Part model, mm, in its own coordinate system. Coordinates: 2 decimals unless noted, no trailing zeros. Order: outer loops, then holes, each group sorted by start corner. A loop starts at its lowest first (then second) coordinate and runs counter-clockwise, first axis right, second up.
1) Mould opens along Y. For faces 1 (the flat face through (24, 10, -4)), 2 (the cylindrical face through (64.851, 7.578, -18.437)), 3 (the cylindrical face through (67.67, 5.78, 10.32)), 4 (the flat face through (24, 5, -19.07)) say: +Y half, -Y half, draft (parallel to the pull), parting line (faces both ways), or undercut.
2) Wall check: L1, parallel to X at y = 5, z = -18.7; L2, parallel to X at y = 6.5, z = 3; L3, parallel to Z at x = 62.5, y = 1.5. Give the ranges that are in metal, low to high.
3) Cut at A-A (y = 5). List the corners of the cut face in (x, z), and give its area (3 significant figures).
4) Cut at C-C (z = -15.5). List the corners of the cut face in (x, y).
5) Pin check, flat tip, straight feed: pin 1 Ø7.5 at (x, z) = (65.19, -11.57) entering from -Y. Stop position of the tip, or through.
6) Cut at B-B (z = -9). List the corners of the cut face in (x, y).
```python
from build123d import *

# Parameters (mm, degrees)
SKETCH1_W           = 100
SKETCH1_H           = 30
SKETCH1_R           = 6.45
BOSS_EXTRUDE1_DEPTH = 10
SKETCH2_R           = 2.6
CUT_EXTRUDE1_DEPTH  = 82.56838771


with BuildPart() as part:
    # Sketch1 → Boss-Extrude1 (new body)
    with BuildSketch(Plane(origin=(0, 0, 0), x_dir=(1, 0, 0), z_dir=(0, 1, 0))):
        with Locations((25.189107413, 4.069591528)):
            Rectangle(SKETCH1_W, SKETCH1_H)
        with Locations(Location((65.189107413, 11.569591528, 0), (0, 0, 270))):
            Circle(SKETCH1_R, mode=Mode.SUBTRACT)
        with Locations(Location((65.189107413, -3.430408472, 0), (0, 0, 270))):
            Circle(SKETCH1_R, mode=Mode.SUBTRACT)
    extrude(amount=BOSS_EXTRUDE1_DEPTH)

    # Sketch2 → Cut-Extrude1 (cut, through all)
    with BuildSketch(Plane.XY.offset(10.930408472)):
        with Locations((65.189107413, 5)):
            Circle(SKETCH2_R)
    extrude(amount=-CUT_EXTRUDE1_DEPTH, mode=Mode.SUBTRACT)


solid = part.part
```
Geometry check:
1. face 1: +Y half
1. face 2: undercut
1. face 3: undercut
1. face 4: draft
2. L1: x = -24.81 to 62.59, 67.79 to 75.19
2. L2: x = -24.81 to 58.75, 71.62 to 75.19
2. L3: z = -19.07 to -17.43, -5.71 to -2.43, 9.29 to 10.93
3. outline: (-24.81, -19.07) - (62.59, -19.07) - (62.59, -17.47) arc R6.45 cw to (62.59, -5.67) - (62.59, -2.47) arc R6.45 cw to (62.59, 9.33) - (62.59, 10.93) - (-24.81, 10.93) - close; (67.79, -19.07) - (75.19, -19.07) - (75.19, 10.93) - (67.79, 10.93) - (67.79, 9.33) arc R6.45 cw to (67.79, -2.47) - (67.79, -5.67) arc R6.45 cw to (67.79, -17.47) - close
3. area: 2,710 mm2
4. outline: (-24.81, 0) - (60.07, 0) - (60.07, 10) - (-24.81, 10) - close; (70.3, 0) - (75.19, 0) - (75.19, 10) - (70.3, 10) - close
5. pin 1: passes through
6. outline: (-24.81, 0) - (59.27, 0) - (59.27, 10) - (-24.81, 10) - close; (71.11, 0) - (75.19, 0) - (75.19, 10) - (71.11, 10) - close
